Check sheet for the modelled part. Datum: model origin and axes. Units: mm. A direction names the side the tool comes from. Give positions to 0.01 mm unless a question says otherwise; leave off trailing zeros. Order: outer loops, then holes, each group sorted by start corner. A loop starts at its lowest first (then second) coordinate and runs counter-clockwise, first axis right, second up.
Item 1: Sectioned sample at A-A on y = -23. Record the boundary of the cut face in (x, z).
Item 2: Access from +Z, -Z, +X, -X, +Y, -Y to the whole of each face (thin tool, end or side, straight path). Record for faces 4 (the flat face through (0, -2.5, -29)), 5 (the flat face through (0, -2.5, 29)), 6 (the flat face through (0, 2.5, 29)).
Item 3: Sectioned sample at B-B on x = -13. Record the boundary of the cut face in (y, z), and give its area (3 significant figures).
Item 4: Release check for a two-part mould opening along Z. For faces 1 (the cylindrical face through (14.4, -7.15, 24.43)), 2 (the flat face through (0, 2.5, -29)), 3 (the cylindrical face through (0.46, -0.04, 30.53)) record: released by +Z, released by -Z, zero draft, split by the parting line, or undercut.
Item 5: Gauge pin test, flat ends, axial feed: P1, Ø6, axis at y = -1.5, z = -31, coming from the +X side; P2, Ø13, axis at x = 3, z = -30.5, coming from the +Y side; P3, Ø1.5, axis at y = 0, z = -30, coming from the -X side; P4, Ø13, axis at x = 2, z = 30, coming from the -Y side. Record the tip position at first contact, or that the pin passes through.
Item 6: Sectioned sample at C-C on z = 17. Record the boundary of the cut face in (x, y).
Item 7: Material ranges on line 1 along Z through (x, y) = (0, 0.6); line 2 along Z through (x, y) = (-5.75, -26.5); line 3 along Y through (x, z) = (-13.5, 11), recorded low to high.
Autodesk Inventor part; units mm, degrees
ref_plane "YZ Plane" through (0, 0, 0) normal (1, 0, 0) x (0, 1, 0)
ref_plane "XZ Plane" through (0, 0, 0) normal (0, 1, 0) x (-1, 0, 0)
ref_plane "XY Plane" through (0, 0, 0) normal (0, 0, 1) x (1, 0, 0)
sketch "Sketch1" plane through (0, 0, 0) normal (0, 1, 0) x (-1, 0, 0)
  line L0 (15, 25) -> (-15, 25)
  line L1 (-15, 25) -> (-15, -25)
  line L2 (-15, -25) -> (15, -25)
  line L3 (15, -25) -> (15, 25)
  circle A0 centre (0, -34) radius 3.5
  arc A1 (-6, -34) -> (6, -34) centre (0, -34) ccw
  line L4 (6, -34) -> (6, -25)
  line L5 (-6, -34) -> (-6, -25)
  line L6 (21.3749, 0) -> (-33.1106, 0) construction
  circle A2 centre (0, 34) radius 3.5
  arc A3 (6, 34) -> (-6, 34) centre (0, 34) ccw
  line L7 (6, 34) -> (6, 25)
  line L8 (-6, 34) -> (-6, 25)
  point P0 (0, 0)
  dimension "d0" = 25
  dimension "d1" = 25
  dimension "d2" = 15
  dimension "d3" = 15
  dimension "d4" = 7
  dimension "d5" = 12
  dimension "d6" = 9
  dimension "d7" = 34
  dimension "d8" = 12
  dimension "d9" = 34
extrude "Extrusion1" add sketch "Sketch1" along normal mid plane 5
sketch "Sketch2" plane through (0, 2.5, 0) normal (0, 1, 0) x (1, 0, 0)
  line L0 (-15, -25) -> (-15, 25)
  line L1 (6, 25) -> (15, 25)
  line L2 (-15, -25) -> (15, -25)
  line L3 (15, -25) -> (15, 25)
  line L4 (15, 25) -> (-15, 25)
  line L5 (-15, 25) -> (-15, -25)
  point P0 (0, 0)
extrude "Extrusion2" add sketch "Sketch2" along normal blind 15 and the other way blind 35
sketch "Sketch3" plane through (0, 17.5, 0) normal (0, 1, 0) x (1, 0, 0)
  circle A0 centre (0, 15) radius 4
  line L0 (15, 25) -> (-15, 25)
  line L1 (-4, 15) -> (-5, 15) construction
  line L2 (-5, 15) -> (-5, 15.5)
  line L3 (-5, 15.5) -> (-3.8219, 16.1802)
  line L4 (-5, 15) -> (-5, 14.5)
  line L5 (-5, 14.5) -> (-3.8219, 13.8198)
  line L6 (-3.8891, 11.818) -> (-3.537, 13.132)
  line L7 (-3.5355, 11.4645) -> (-3.8891, 11.818)
  line L8 (-3.5355, 11.4645) -> (-3.182, 11.1109)
  line L9 (-3.182, 11.1109) -> (-1.868, 11.463)
  line L10 (-0.5, 10) -> (-1.1802, 11.1781)
  line L11 (0, 10) -> (-0.5, 10)
  line L12 (0, 10) -> (0.5, 10)
  line L13 (0.5, 10) -> (1.1802, 11.1781)
  line L14 (3.182, 11.1109) -> (1.868, 11.463)
  line L15 (3.5355, 11.4645) -> (3.182, 11.1109)
  line L16 (3.5355, 11.4645) -> (3.8891, 11.818)
  line L17 (3.8891, 11.818) -> (3.537, 13.132)
  line L18 (5, 14.5) -> (3.8219, 13.8198)
  line L19 (5, 15) -> (5, 14.5)
  line L20 (5, 15) -> (5, 15.5)
  line L21 (5, 15.5) -> (3.8219, 16.1802)
  line L22 (3.8891, 18.182) -> (3.537, 16.868)
  line L23 (3.5355, 18.5355) -> (3.8891, 18.182)
  line L24 (3.5355, 18.5355) -> (3.182, 18.8891)
  line L25 (3.182, 18.8891) -> (1.868, 18.537)
  line L26 (0.5, 20) -> (1.1802, 18.8219)
  line L27 (0, 20) -> (0.5, 20)
  line L28 (0, 20) -> (-0.5, 20)
  line L29 (-0.5, 20) -> (-1.1802, 18.8219)
  line L30 (-3.182, 18.8891) -> (-1.868, 18.537)
  line L31 (-3.5355, 18.5355) -> (-3.182, 18.8891)
  line L32 (-3.5355, 18.5355) -> (-3.8891, 18.182)
  line L33 (-3.8891, 18.182) -> (-3.537, 16.868)
  point P0 (0, 0)
  dimension "d16" = 8
  dimension "d17" = 10
  dimension "d18" = 15
  dimension "d19" = 120
  dimension "d20" = 0
  dimension "d21" = 1
  dimension "d22" = 0.5
  dimension "d25" = 360
extrude "Extrusion3" add sketch "Sketch3" along normal blind 10
fillet "Fillet1" radius 2 2 edges at (15, -7.5, 25) (15, -7.5, -25)
thread "Thread1"
thread "Thread2"
properties part number "servo" material "Rubber"
Report:
1. outline: (-15, -25) - (13, -25) arc R2 ccw to (15, -23) - (15, 23) arc R2 ccw to (13, 25) - (-15, 25) - close
2. face 4: -Z, +X, -X, -Y
2. face 5: +Z, +X, -X, -Y
2. face 6: +Z, +X, -X, +Y
3. outline: (-32.5, -25) - (17.5, -25) - (17.5, 25) - (-32.5, 25) - close
3. area: 2,500 mm2
4. face 1: released by +Z
4. face 2: zero draft
4. face 3: undercut
5. P1: stops at x = 6
5. P2: stops at y = 17.5
5. P3: stops at x = -6
5. P4: stops at y = -32.5
6. outline: (-15, -32.5) - (15, -32.5) - (15, 17.5) - (-15, 17.5) - close
7. line 1: z = -40 to -37.5, -30.5 to 30.5, 37.5 to 40
7. line 2: z = -25 to 25
7. line 3: y = -32.5 to 17.5
